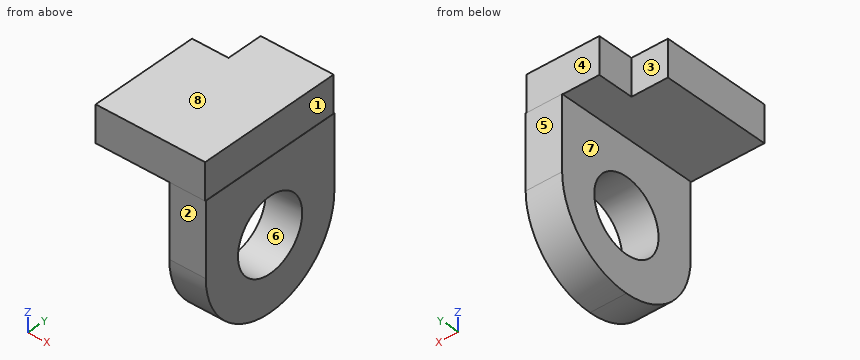
from build123d import *

# Parameters (mm, degrees)
F1_DEPTH = 12.7
F2_W     = 12.7
F2_H     = 50.8
F3_DEPTH = 50.8
F4_R     = 12.7
F5_DEPTH = 21.59
F7_DEPTH = 25.4


with BuildPart() as f1:
    # F0 (on Top) → F1 (new body)
    with BuildSketch(Plane.XY):
        Polygon((19.05, -25.4), (19.05, 25.4), (-6.35, 25.4), (-6.35, 12.7), (-19.05, 12.7), (-19.05, -25.4), align=None)
    extrude(amount=F1_DEPTH)

    # F2 (on Top) → F3 (join)
    with BuildSketch(Plane.XY):
        with Locations((12.775489, 0.181956)):
            Rectangle(F2_W, F2_H)
    extrude(amount=-F3_DEPTH)

    # F4 (on Right) → F5 (cut)
    with BuildSketch(Plane.YZ):
        with Locations((0.181956, -25.4)):
            Circle(F4_R)
    extrude(amount=F5_DEPTH, mode=Mode.SUBTRACT)

    # F6 (on face) → F7 (cut)
    with BuildSketch(Plane(origin=(6.425489, 0, 0), x_dir=(0, -1, 0), z_dir=(-1, 0, 0))):
        with BuildLine():
            ThreePointArc((25.218044, -25.4), (17.778556, -43.360512), (-0.181956, -50.8))
            Line((-0.181956, -50.8), (25.218044, -50.8))
            Line((25.218044, -50.8), (25.218044, -25.4))
        make_face()
        with BuildLine():
            ThreePointArc((-0.181956, -50.8), (-18.142468, -43.360512), (-25.581956, -25.4))
            Line((-25.581956, -25.4), (-25.581956, -50.8))
            Line((-25.581956, -50.8), (-0.181956, -50.8))
        make_face()
    extrude(amount=-F7_DEPTH, mode=Mode.SUBTRACT)


solid = f1.part
For this review, take the finished solid that the model builds, in its own axes (mm). Face numbers are marked on the shaded views. A direction names the side the tool comes from. Give positions to 0.01 mm unless a question says otherwise; leave off trailing zeros. Loops run counter-clockwise (first coordinate to the right, second up) from the corner with the lowest first, then second, coordinate; pieces in that order, holes last. Notation, with made-up numbers: M -38,59 L -34,59 A25 ccw -34,75 Z; hole C 58.25,57 d1. An arc over 180 degrees is marked long. Answer as a JSON object with one key per item and string values. Group by question number.
Q1. Tool access review of the marked faces 1, 2, 3, 4 and 5: name each direction out of +Z, -Z, +X, -X, +Y, -Y from which nothing blocks a thin tool from reaching the whole face with its end or side.
Q2. Mouldability with a two-part tool opening along Z and no side actions: class the marked faces 6, 7 and 8 as +Z half, -Z half, draft (parallel to the pull), parting line (faces both ways), or undercut.
Q3. For probe 1 along Y at (x, z) = (13, -25); probe 2 along X at (y, z) = (19, -21.5); probe 3 along Z at (x, y) = (-13, 6.5), list the stretches that pass through material, from the lowest coordinate up. Write a range as [from, to].
Q4. Add section C-C on x = -12.5. Give the boundary of the cut face in (y, z), and give its area (3 significant figures).
Q5. Insertion check: P1, Ø15, axis at y = 4.5, z = -13.5, coming from the -X side; P2, Ø2, axis at x = 5, z = -23, coming from the +Y side; P3, Ø4, axis at y = 20, z = 5.5, coming from the -X side; P4, Ø6.5, axis at x = 10, z = 6, coming from the +Y side. Each pin has a flat end and moves straight along its axis. Give the tip position at first contact, or say it passes through.
Q6. Add section B-B on y = 19. Give the boundary of the cut face in (x, z).
Q7. Add section A-A on z = -10.5. Give the boundary of the cut face in (x, y).
Q8. Add section D-D on z = 8. Give the boundary of the cut face in (x, y).
Checked values:
{
 "1": {"face 1": "+Z, +X, +Y, -Y", "face 2": "-Z, +X, -X, -Y", "face 3": "+Z, -Z, -X, +Y", "face 4": "+Z, +X, -X, +Y", "face 5": "+Z, -Z, +X, -X, +Y"},
 "2": {"face 6": "undercut", "face 7": "draft", "face 8": "+Z half"},
 "3": {"probe 1": "[-25.22, -12.51], [12.88, 25.58]", "probe 2": "[6.43, 19.13]", "probe 3": "[0, 12.7]"},
 "4": {"outline": "M -25.4,0 L 12.7,0 L 12.7,12.7 L -25.4,12.7 Z", "area": "484 mm²"},
 "5": {"P1": "x = 6.43", "P2": "through", "P3": "x = -6.35", "P4": "y = 25.4"},
 "6": {"outline": "M -6.35,0 L 6.43,0 L 6.43,-42.46 L 19.13,-42.46 L 19.13,0 L 19.05,0 L 19.05,12.7 L -6.35,12.7 Z"},
 "7": {"outline": "M 6.43,-25.22 L 19.13,-25.22 L 19.13,25.58 L 6.43,25.58 Z"},
 "8": {"outline": "M -19.05,-25.4 L 19.05,-25.4 L 19.05,25.4 L -6.35,25.4 L -6.35,12.7 L -19.05,12.7 Z"}
}
